Source: CAD feature listing. Evaluate the final solid. Frame: model axes, mm. Face numbers are marked on the shaded views. A direction names the side the tool comes from. Give positions to 0.01 mm unless a question says otherwise; leave off trailing zeros. Write each loop counter-clockwise with the first axis right and the second up, starting at its lowest first coordinate (ties: lowest second). Pieces come first, ordered by that corner, then holes. Notation, with made-up numbers: (58.5, 41.25) - (104.5, 41.25) arc R25 cw to (104.5, 53.25) - close; hole circle Ø1 at (54.25, 57). An arc over 180 degrees is marked (long way). Answer as a JSON object with one key per item and string values. Group by question number.
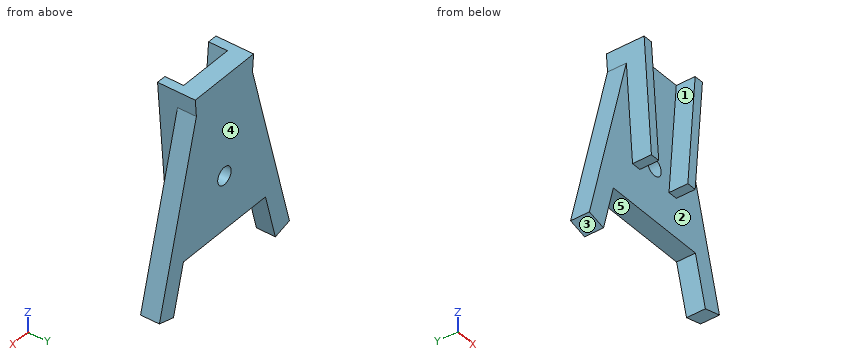
Autodesk Inventor part; units mm, degrees
ref_plane "YZ Plane" through (0, 0, 0) normal (1, 0, 0) x (0, 1, 0)
ref_plane "XZ Plane" through (0, 0, 0) normal (0, 1, 0) x (-1, 0, 0)
ref_plane "XY Plane" through (0, 0, 0) normal (0, 0, 1) x (1, 0, 0)
sketch "Sketch1" plane through (0, 0, 0) normal (0, 1, 0) x (-1, 0, 0)
  circle A0 centre (0, 0) radius 0.5
  line L0 (0, 0) -> (0, -2)
  circle A1 centre (0, -2) radius 0.75
  line L1 (0, -2) -> (0, -4)
  line L2 (0, -4) -> (0, -6)
  circle A2 centre (0, -4) radius 0.5
  circle A3 centre (0, -6) radius 0.5
  line L3 (0, 1.25) -> (0, 0)
  line L4 (0, 0.5) -> (0, 4.8)
  line L5 (0, 4.8) -> (0, -22.2)
  line L6 (0, -6.5) -> (0, -8)
  line L7 (0, -6) -> (0, -8)
  circle A4 centre (0, -8) radius 0.5
  line L8 (0, -8.5) -> (0, -12.5)
  line L9 (0, -12.5) -> (0, -12)
  circle A5 centre (0, -10.5) radius 0.925
  circle A6 centre (0, -12) radius 0.5
  line L10 (0, 1.25) -> (3, 1.25)
  line L11 (3, 1.25) -> (-3, 1.25)
  line L12 (-3, 1.25) -> (-3, -13.75)
  line L13 (-3, -13.75) -> (3, -13.75)
  line L14 (3, -13.75) -> (3, 1.25)
  line L15 (3, 0) -> (-3, 0)
  line L16 (0, -12) -> (2, -12)
  line L17 (2, -12) -> (-2, -12)
  line L18 (-2, -12) -> (-3, 0)
  line L19 (2, -12) -> (3, 0)
  line L20 (3, 0) -> (4, 0)
  line L21 (2, -12) -> (3, -12)
  line L22 (3, -12) -> (4, 0)
  line L23 (-3, 0) -> (-4, 0)
  line L24 (-2, -12) -> (-3, -12)
  line L25 (-4, 0) -> (-3, -12)
  line L26 (0, 4.8) -> (6.9881, -21.28)
  line L27 (0, 4.8) -> (-6.9881, -21.28)
  line L28 (-6.9881, -21.28) -> (-8.9881, -21.28)
  line L29 (-6.9881, -21.28) -> (-8.92, -20.7624)
  line L30 (-8.92, -20.7624) -> (-8.92, -1.1218)
  line L31 (-8.92, -20.7624) -> (-3.8366, -1.791)
  line L32 (6.9881, -21.28) -> (8.9881, -21.28)
  line L33 (6.9881, -21.28) -> (8.92, -20.7624)
  line L34 (8.92, -20.7624) -> (8.92, -0.4933)
  line L35 (8.92, -20.7624) -> (3.674, -1.184)
  line L36 (0, -22.2) -> (0, -16.2)
  line L37 (0, -16.2) -> (5.6269, -16.2)
  line L38 (0, -16.2) -> (-5.6269, -16.2)
  point P0 (0, -11.5)
  point P1 (3.8474, -1.8313)
  point P2 (-3.8474, -1.8313)
  dimension "d0" = 1
  dimension "d6" = 1
  dimension "d42" = 1
  dimension "d1" = 2
  dimension "d2" = 1.5
  dimension "d3" = 2
  dimension "d4" = 2
  dimension "d5" = 1
  dimension "d10" = 1.25
  dimension "d13" = 4.3
  dimension "d16" = 27
  dimension "d41" = 2
  dimension "d43" = 4
  dimension "d44" = 0.5
  dimension "d45" = 1
  dimension "d46" = 1.85
  dimension "d47" = 3
  dimension "d48" = 6
  dimension "d49" = 15
  dimension "d61" = 2
  dimension "d62" = 4
  dimension "d63" = 1
  dimension "d64" = 1
  dimension "d65" = 1
  dimension "d66" = 1
  dimension "d69" = 2
  dimension "d70" = 27
  dimension "d71" = 27
  dimension "d72" = 2
  dimension "d73" = 2
  dimension "d75" = 2
  dimension "d76" = 2
  dimension "d77" = 6
extrude "Extrusion1" add sketch "Sketch1" along normal blind 2 contours L15 L26 L19 L16 A6 L5 A5 A4 A3 L2 A2 L1 A1 L0 A0 | A0 L0 L15 | L0 A1 L1 A2 L2 A3 L5 A4 A5 A6 L17 L18 L27 L15 A0 | A0 L15 L0 | L15 L19 L26 | A1 L1 L0 | L0 L1 A1 | L20 L22 L26 L14 | L14 L26 L19 | L26 L14 L21 L19 | L27 L18 L15 | L26 L22 L14 | L21 L14 L13 L5 A6 L16 | L18 L27 L12 | L12 L27 L25 L23 | L18 L24 L12 L27 | A2 L2 L1 | L1 L2 A2 | L22 L26 L37 L5 L13 L14 | L22 L35 L33 L26 | L16 L5 A6 | A6 L5 L16 | L12 L25 L27 | L17 A6 L5 L13 L12 L24 | A6 L17 L5 | L5 L17 A6 | L12 L13 L5 L38 L27 L25 | L27 L29 L31 L25 | A3 L5 L2 | L2 L5 A3 | A4 L5 | L5 A4
extrude "Extrusion2" add sketch "Sketch1" against normal blind 2 contours L20 L22 L26 L14 | L14 L26 L19 | L26 L14 L21 L19 | L26 L22 L14 | L18 L27 L12 | L12 L27 L25 L23 | L18 L24 L12 L27 | L12 L25 L27
properties part number "Servo Arm"
Q1. First-contact query: pin 1 Ø1.5 at (y, z) = (-1, -3.5) entering from +X; pin 2 Ø0.5 at (x, y) = (2.5, -1.5) entering from -Z; pin 3 Ø0.6 at (x, y) = (2, 1.5) entering from -Z. Flat tips, straight axial feed; report the tip coordinate or a pass-through.
Q2. Section D-D on z = -5.75. Return the cut outline in (x, y), then the cut area to 3 significant figures.
Q3. Ray query, probe 1 along Z at (x, y) = (0, 1.3) (3 decimals); probe 2 along X at (y, z) = (0.9, -10.5) (3 decimals); probe 3 along Y at (x, z) = (-8, -19.5). Return the intervals inside material, ascending. Write a range as [from, to].
Q4. Reachability of the marked faces 4 and 5 from +Z, -Z, +X, -X, +Y, -Y: full face, straight path, thin tool, end or side. Return the list, or none.
Q5. Section C-C on y = 1.45. Return the cut outline in (x, z) (3 decimals).
Q6. Section A-A on x = 0. Return the cut outline in (y, z) (3 decimals), then the cut area to 3 significant figures.
Q7. Section B-B on z = -10.5. Return the cut outline in (x, y) (3 decimals), then the cut area to 3 significant figures.
Q8. Draft query along Z for the marked faces 1, 2 and 3. Return one class per face: released by +Z, released by -Z, zero draft, split by the parting line, or undercut.
Taken from the geometry:
{
 "1": {"pin 1": "stops at x = 3.77", "pin 2": "stops at z = -12", "pin 3": "stops at z = -16.2"},
 "2": {"outline": "(-4.9, 0) - (-3.52, 0) - (-3.52, -2) - (-2.52, -2) - (-2.52, 0) - (2.52, 0) - (2.52, -2) - (3.52, -2) - (3.52, 0) - (4.9, 0) - (4.9, 2) - (-4.9, 2) - close", "area": "23.6 mm²"},
 "3": {"probe 1": "z = [-16.2, -11.425], [-9.575, 0]", "probe 2": "x = [-6.17, -0.925], [0.925, 6.17]", "probe 3": "y = [0, 2]"},
 "4": {"face 4": "+Z, -Z, +X, -X, +Y", "face 5": "-Z, +Y, -Y"},
 "5": {"outline": "(-8.92, -20.762) - (-6.988, -21.28) - (-5.627, -16.2) - (5.627, -16.2) - (6.988, -21.28) - (8.92, -20.762) - (3.847, -1.831) - (4, 0) - (-4, 0) - (-3.847, -1.831) - close; hole circle Ø1.85 at (0, -10.5)"},
 "6": {"outline": "(0, -16.2) - (2, -16.2) - (2, -11.425) - (0, -11.425) - close; (0, -9.575) - (2, -9.575) - (2, 0) - (0, 0) - close", "area": "28.7 mm²"},
 "7": {"outline": "(-6.17, 0) - (-3.125, 0) - (-3.125, -2) - (-2.125, -2) - (-2.125, 0) - (-0.925, 0) - (-0.925, 2) - (-6.17, 2) - close; (0.925, 0) - (2.125, 0) - (2.125, -2) - (3.125, -2) - (3.125, 0) - (6.17, 0) - (6.17, 2) - (0.925, 2) - close", "area": "25.0 mm²"},
 "8": {"face 1": "released by +Z", "face 2": "zero draft", "face 3": "released by -Z"}
}
